Geometry: see drawing. Coordinates: mm, zero at the bounding-box minimum. Round coordinates to 2 decimals unless told otherwise and drop trailing zeros. Loops run counter-clockwise (first coordinate to the right, second up) from the corner with the lowest first, then second, coordinate; pieces in that order, holes last.
(1) Section D-D, the plane y = 2.05. Count the separate pieces of the cut face and the enclosed holes in it.
(2) Section A-A, the plane z = 96.5. Return the cut outline in (x, y).
(3) Material intervals for probe 1 along X at (y, z) = (2.75, 75); probe 2 along X at (y, z) = (2.4, 12); probe 3 along Z at (x, y) = (116, 0.85) (1 decimal), sorted ascending.
(4) Section B-B, the plane z = 12. Return the cut outline in (x, y).
(5) Section C-C, the plane x = 118.5. Return the cut outline in (y, z) (1 decimal).
(6) First-contact query: pin 1 Ø2.5 at (y, z) = (2.5, 1) entering from -X. Flat tip, straight axial feed; report the tip coordinate or a pass-through.
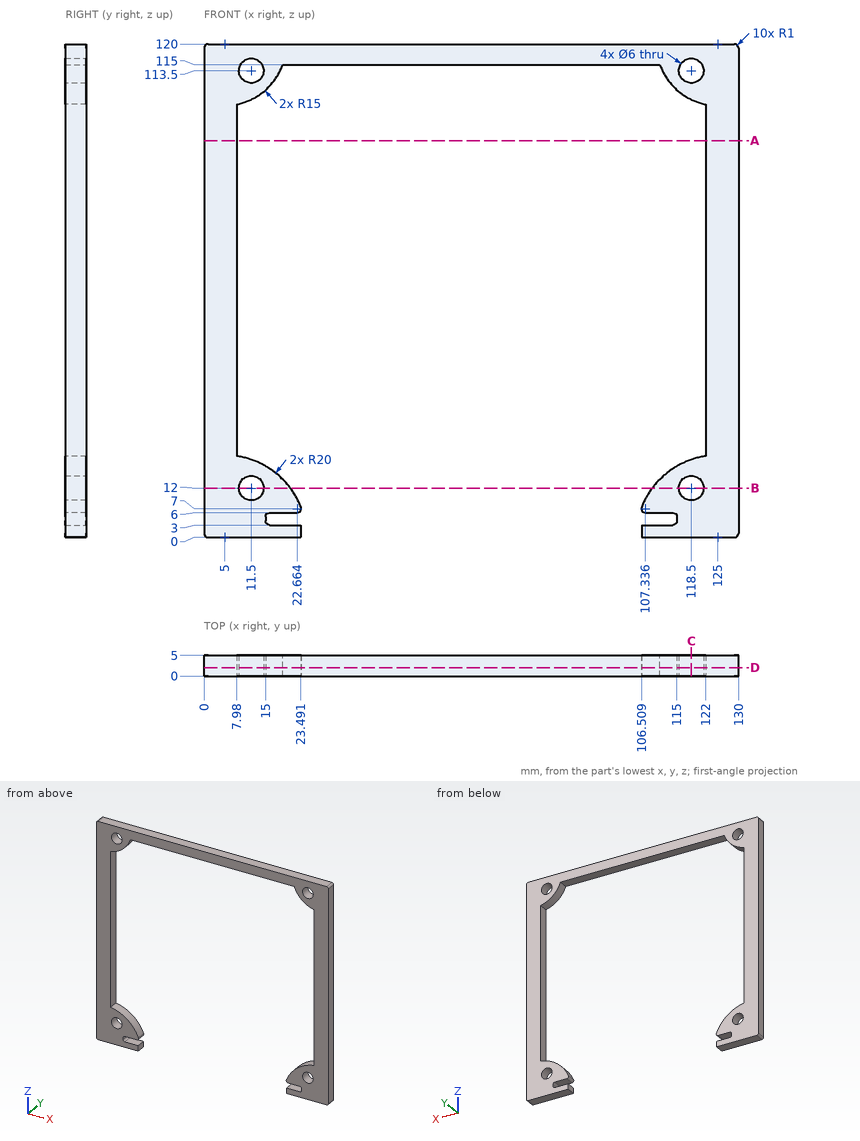
Output values:
1. separate pieces: 1
1. enclosed holes: 4
2. outline: (0, 0) - (7.98, 0) - (7.98, 5) - (0, 5) - close; (122, 0) - (130, 0) - (130, 5) - (122, 5) - close
3. probe 1: x = 0 to 7.98, 122 to 130
3. probe 2: x = 0 to 8.5, 14.5 to 21, 109 to 115.5, 121.5 to 130
3. probe 3: z = 0 to 10.3, 13.7 to 17.9, 108 to 111.8, 115.2 to 120
4. outline: (0, 0) - (8.5, 0) - (8.5, 5) - (0, 5) - close; (14.5, 0) - (21, 0) - (21, 5) - (14.5, 5) - close; (109, 0) - (115.5, 0) - (115.5, 5) - (109, 5) - close; (121.5, 0) - (130, 0) - (130, 5) - (121.5, 5) - close
5. outline: (0, 0) - (5, 0) - (5, 9) - (0, 9) - close; (0, 15) - (5, 15) - (5, 18.9) - (0, 18.9) - close; (0, 106.5) - (5, 106.5) - (5, 110.5) - (0, 110.5) - close; (0, 116.5) - (5, 116.5) - (5, 120) - (0, 120) - close
6. pin 1: stops at x = 0
